```python
from build123d import *

# Parameters (mm, degrees)
BOSS_EXTRUDE1_DEPTH = 3.175
SKETCH2_R           = 1.4732
CUT_EXTRUDE1_DEPTH  = 4.175
FILLET1_R           = 3
FILLET3_R           = 2


with BuildPart() as part:
    # Sketch1 → Boss-Extrude1 (new body)
    with BuildSketch(Plane.XY):
        with BuildLine():
            Line((-17.122741189, 26.5), (-17.122741189, 44.5))
            Line((-17.122741189, 44.5), (-47.122741189, 44.5))
            ThreePointArc((-47.122741189, 44.5), (-58.300369938, 30.054224058), (-64.75017234, 12.965635))
            Line((-64.75017234, 12.965635), (-58.20928788, 12.965635))
            ThreePointArc((-58.20928788, 12.965635), (-56.652290629, 18.243467198), (-54.577718421, 23.340123288))
            ThreePointArc((-54.577718421, 23.340123288), (-35.916757127, 25.708630171), (-17.122741189, 26.5))
        make_face()
    extrude(amount=BOSS_EXTRUDE1_DEPTH)

    # Sketch2 → Cut-Extrude1 (cut, through all)
    with BuildSketch(Plane.XY.offset(3.175)):
        with Locations((-20.889565657, 40.81189221)):
            Circle(SKETCH2_R)
        with Locations((-39.939565657, 40.81189221)):
            Circle(SKETCH2_R)
    extrude(amount=-CUT_EXTRUDE1_DEPTH, mode=Mode.SUBTRACT)

    # Fillet1
    fillet1_edges = [part.edges().sort_by_distance(p)[0] for p in [
        (-47.122741189, 44.5, 1.5875),
        (-17.122741189, 44.5, 1.5875),
        (-17.122741189, 26.5, 1.5875),
        (-54.577718421, 23.340123288, 1.5875),
    ]]
    fillet(fillet1_edges, radius=FILLET1_R)

    # Fillet3
    fillet3_edges = [part.edges().sort_by_distance(p)[0] for p in [
        (-58.20928788, 12.965635, 1.5875),
        (-64.75017234, 12.965635, 1.5875),
    ]]
    fillet(fillet3_edges, radius=FILLET3_R)


solid = part.part
```
Can you work these out from the model? Positions are in its coordinate system, mm. Round coordinates to 2 decimals unless told otherwise and drop trailing zeros. Loops run counter-clockwise (first coordinate to the right, second up) from the corner with the lowest first, then second, coordinate; pieces in that order, holes last. Notation, with made-up numbers: M -0.5,83.25 L 34.5,83.25 A29 ccw 34.5,108.25 Z; hole C 26.5,12.25 d7. An arc over 180 degrees is marked long. Answer in a Markdown table with one row per item.
1. If we section it at C-C, the plane x = -29: Please give me the cut outline in (y, z) (3 decimals).
Established:
| item | result |
|---|---|
| outline | M 26.184,0 L 44.5,0 L 44.5,3.175 L 26.184,3.175 Z |
2. Please list where these lines run through material, in increasing order: line 1 (Y direction, x = -40, z = 1.35); line 2 (Y direction, x = -35, z = 0.7); line 3 (X direction, y = 33, z = 2.3). Write a range as from..to.
Established:
| item | result |
|---|---|
| line 1 | 25.33..39.34, 42.28..44.5 |
| line 2 | 25.78..44.5 |
| line 3 | -56.54..-17.12 |
3. I'm going to push a flat-ended pin straight in: pin 1 Ø1 at (x, z) = (-58, 1.5) entering from -Y. Where does the tip first touch, or does it pass through?
Established:
| item | result |
|---|---|
| pin 1 | y = 13.41 |
4. Thinking about a two-plate mould opening in X: for faces 1 (the face through (-63.818, 13.762, 1.61)), 2 (the face through (-41, 32, 3.175)), 3 (the face through (-41.025, 41.808, 1.61)), which applies, pulls with the +X half, pulls with the -X half, needs draft (parallel to the pull), parting line crosses it, or undercut?
Established:
| item | result |
|---|---|
| face 1 | pulls with the -X half |
| face 2 | needs draft |
| face 3 | undercut |
5. If we section it at B-B, the plane y = 35: Please give me the cut outline in (x, z) (3 decimals).
Established:
| item | result |
|---|---|
| outline | M -55.22,0 L -17.123,0 L -17.123,3.175 L -55.22,3.175 Z |
6. If we section it at A-A, the plane z = 2.6: Give the number of separate pieces and of enclosed holes in the cut face, plus the area to 3 significant figures.
Established:
| item | result |
|---|---|
| separate pieces | 1 |
| enclosed holes | 2 |
| area | 782 mm² |
